Input: part model. Units: mm. Frame: model coordinates. Face numbers are marked on the shaded views. A direction names the side the tool comes from. Give positions to 0.01 mm unless a question says otherwise; leave off trailing zeros. Loops run counter-clockwise (first coordinate to the right, second up) from the corner with the lowest first, then second, coordinate; pieces in that order, holes last. Notation, with made-up numbers: (68.5, 24.25) - (73.5, 24.25) arc R28 ccw to (73.5, 56.25) - close; hole circle Ø1 at (44, 19). An arc over 180 degrees is marked (long way). One line per item, written item: value.
from build123d import *
from build123d.topology import SkipClean

# Parameters (mm, degrees)
SKETCH1_R                                           = 12
SKETCH1_R_2                                         = 2
SQUARE_BODY_DEPTH                                   = 11
CBORE_FOR_0_BINDING_HEAD_MACHINE_SCREW1_D           = 1.778
CBORE_FOR_0_BINDING_HEAD_MACHINE_SCREW1_CBORE_D     = 3.97002
CBORE_FOR_0_BINDING_HEAD_MACHINE_SCREW1_CBORE_DEPTH = 4.812792
CBORE_FOR_0_BINDING_HEAD_MACHINE_SC_2_D             = 1.778
CBORE_FOR_0_BINDING_HEAD_MACHINE_SC_2_CBORE_D       = 3.97002
CBORE_FOR_0_BINDING_HEAD_MACHINE_SC_2_CBORE_DEPTH   = 4.812792
F_6_32_TAPPED_HOLE2_D                               = 2.7051
F_6_32_TAPPED_HOLE2_DEPTH                           = 10.5
CENTER_SPINDLE_DEPTH                                = 21.223748416
SKETCH1_3_R                                         = 14
SKETCH1_3_R_2                                       = 12
TOP_FLANGE_DEPTH                                    = 2
BOTTOM_START                                        = 9
SKETCH1_4_R                                         = 14
SKETCH1_4_R_2                                       = 12
BOTTOM_FLANGE_DEPTH                                 = 2


with BuildPart() as part:
    # Sketch1 → Square Body (new body)
    # profile 1 of 10: a face of its own
    with BuildSketch(Plane.XY):
        Circle(SKETCH1_R)
        Circle(SKETCH1_R_2, mode=Mode.SUBTRACT)
    # profile 2 of 10: a face of its own
    with BuildSketch(Plane.XY):
        with BuildLine():
            Line((-12, 7.211102551), (-12, 0))
            ThreePointArc((-12, 0), (-8.485281374, 8.485281374), (0, 12))
            Line((0, 12), (-7.211102551, 12))
            ThreePointArc((-7.211102551, 12), (-9.899494937, 9.899494937), (-12, 7.211102551))
        make_face()
    # profile 3 of 10: a face of its own
    with BuildSketch(Plane.XY):
        with BuildLine():
            Line((-12, 12), (-12, 7.211102551))
            ThreePointArc((-12, 7.211102551), (-9.899494937, 9.899494937), (-7.211102551, 12))
            Line((-7.211102551, 12), (-12, 12))
        make_face()
    # profile 4 of 10: a face of its own
    with BuildSketch(Plane.XY):
        with BuildLine():
            ThreePointArc((0, -12), (-8.485281374, -8.485281374), (-12, 0))
            Line((-12, 0), (-12, -7.211102551))
            ThreePointArc((-12, -7.211102551), (-9.899494937, -9.899494937), (-7.211102551, -12))
            Line((-7.211102551, -12), (0, -12))
        make_face()
    # profile 5 of 10: a face of its own
    with BuildSketch(Plane.XY):
        with BuildLine():
            ThreePointArc((-7.211102551, -12), (-9.899494937, -9.899494937), (-12, -7.211102551))
            Line((-12, -7.211102551), (-12, -12))
            Line((-12, -12), (-7.211102551, -12))
        make_face()
    # profile 6 of 10: a face of its own
    with BuildSketch(Plane.XY):
        with BuildLine():
            ThreePointArc((12, 0), (8.485281374, -8.485281374), (0, -12))
            Line((0, -12), (7.211102551, -12))
            ThreePointArc((7.211102551, -12), (9.899494937, -9.899494937), (12, -7.211102551))
            Line((12, -7.211102551), (12, 0))
        make_face()
    # profile 7 of 10: a face of its own
    with BuildSketch(Plane.XY):
        with BuildLine():
            ThreePointArc((12, -7.211102551), (9.899494937, -9.899494937), (7.211102551, -12))
            Line((7.211102551, -12), (12, -12))
            Line((12, -12), (12, -7.211102551))
        make_face()
    # profile 8 of 10: a face of its own
    with BuildSketch(Plane.XY):
        with BuildLine():
            Line((7.211102551, 12), (0, 12))
            ThreePointArc((0, 12), (8.485281374, 8.485281374), (12, 0))
            Line((12, 0), (12, 7.211102551))
            ThreePointArc((12, 7.211102551), (9.899494937, 9.899494937), (7.211102551, 12))
        make_face()
    # profile 9 of 10: a face of its own
    with BuildSketch(Plane.XY):
        with BuildLine():
            Line((12, 12), (7.211102551, 12))
            ThreePointArc((7.211102551, 12), (9.899494937, 9.899494937), (12, 7.211102551))
            Line((12, 7.211102551), (12, 12))
        make_face()
    # profile 10 of 10: a face of its own
    with BuildSketch(Plane.XY):
        with BuildLine():
            ThreePointArc((2, 0), (1.870828693, 0.707106781), (1.5, 1.322875656))
            Line((1.5, 1.322875656), (1.5, -1.322875656))
            ThreePointArc((1.5, -1.322875656), (1.870828693, -0.707106781), (2, 0))
        make_face()
    extrude(amount=SQUARE_BODY_DEPTH)

    # CBORE for #0 Binding Head Machine Screw1 (through all)
    with Locations(Plane(origin=(-12, 7.5, 5.85), x_dir=(0, -1, 0), z_dir=(-1, 0, 0))):
        with Locations((0, 0)):
            CounterBoreHole(CBORE_FOR_0_BINDING_HEAD_MACHINE_SCREW1_D / 2, CBORE_FOR_0_BINDING_HEAD_MACHINE_SCREW1_CBORE_D / 2, CBORE_FOR_0_BINDING_HEAD_MACHINE_SCREW1_CBORE_DEPTH)

    # CBORE for _0 Binding Head Machine Sc 2 (through all)
    with Locations(Plane(origin=(12, -7.5, 5.85), x_dir=(0, 0, 1), z_dir=(1, 0, 0))):
        with Locations((0, 0)):
            CounterBoreHole(CBORE_FOR_0_BINDING_HEAD_MACHINE_SC_2_D / 2, CBORE_FOR_0_BINDING_HEAD_MACHINE_SC_2_CBORE_D / 2, CBORE_FOR_0_BINDING_HEAD_MACHINE_SC_2_CBORE_DEPTH)

    # #6-32 Tapped Hole2
    with Locations(Plane(origin=(12, 0, 5.85), x_dir=(0, 1, 0), z_dir=(1, 0, 0))):
        with Locations((0, 0)):
            Hole(F_6_32_TAPPED_HOLE2_D / 2, depth=F_6_32_TAPPED_HOLE2_DEPTH)

    # Sketch1<5> → Center Spindle (cut, through all)
    with SkipClean():  # the faces are left unmerged after this step: merging them gives an invalid solid
        with BuildSketch(Plane.XY):
            with BuildLine():
                ThreePointArc((0, -12), (-8.485281374, -8.485281374), (-12, 0))
                Line((-12, 0), (-12, -7.211102551))
                ThreePointArc((-12, -7.211102551), (-9.899494937, -9.899494937), (-7.211102551, -12))
                Line((-7.211102551, -12), (0, -12))
            make_face()
            with BuildLine():
                ThreePointArc((-7.211102551, -12), (-9.899494937, -9.899494937), (-12, -7.211102551))
                Line((-12, -7.211102551), (-12, -12))
                Line((-12, -12), (-7.211102551, -12))
            make_face()
            with BuildLine():
                Line((-12, 7.211102551), (-12, 0))
                ThreePointArc((-12, 0), (-8.485281374, 8.485281374), (0, 12))
                Line((0, 12), (-7.211102551, 12))
                ThreePointArc((-7.211102551, 12), (-9.899494937, 9.899494937), (-12, 7.211102551))
            make_face()
            with BuildLine():
                Line((-12, 12), (-12, 7.211102551))
                ThreePointArc((-12, 7.211102551), (-9.899494937, 9.899494937), (-7.211102551, 12))
                Line((-7.211102551, 12), (-12, 12))
            make_face()
            with BuildLine():
                Line((7.211102551, 12), (0, 12))
                ThreePointArc((0, 12), (8.485281374, 8.485281374), (12, 0))
                Line((12, 0), (12, 7.211102551))
                ThreePointArc((12, 7.211102551), (9.899494937, 9.899494937), (7.211102551, 12))
            make_face()
            with BuildLine():
                Line((12, 12), (7.211102551, 12))
                ThreePointArc((7.211102551, 12), (9.899494937, 9.899494937), (12, 7.211102551))
                Line((12, 7.211102551), (12, 12))
            make_face()
            with BuildLine():
                ThreePointArc((12, 0), (8.485281374, -8.485281374), (0, -12))
                Line((0, -12), (7.211102551, -12))
                ThreePointArc((7.211102551, -12), (9.899494937, -9.899494937), (12, -7.211102551))
                Line((12, -7.211102551), (12, 0))
            make_face()
            with BuildLine():
                ThreePointArc((12, -7.211102551), (9.899494937, -9.899494937), (7.211102551, -12))
                Line((7.211102551, -12), (12, -12))
                Line((12, -12), (12, -7.211102551))
            make_face()
        extrude(amount=CENTER_SPINDLE_DEPTH, mode=Mode.SUBTRACT)

    # Sketch1<3> → Top Flange (add)
    with SkipClean():  # the faces are left unmerged after this step: merging them gives an invalid solid
        with BuildSketch(Plane.XY):
            Circle(SKETCH1_3_R)
            Circle(SKETCH1_3_R_2, mode=Mode.SUBTRACT)
        extrude(amount=TOP_FLANGE_DEPTH)

    # Sketch1<4> → Bottom Flange (add)
    with SkipClean():  # the faces are left unmerged after this step: merging them gives an invalid solid
        with BuildSketch(Plane.XY.offset(BOTTOM_START)):
            Circle(SKETCH1_4_R)
            Circle(SKETCH1_4_R_2, mode=Mode.SUBTRACT)
        extrude(amount=BOTTOM_FLANGE_DEPTH)


solid = part.part
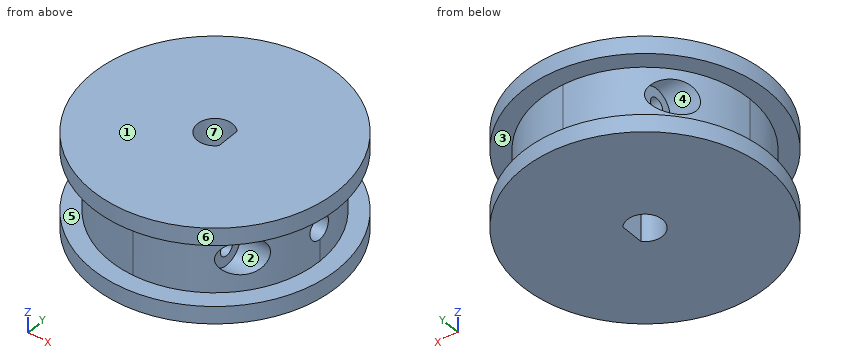
Item 1: Draft query along X for the marked faces 5, 6 and 7. Return one class per face: pulls with the +X half, pulls with the -X half, needs draft (parallel to the pull), parting line crosses it, or undercut.
Verdict:
face 5: needs draft
face 6: parting line crosses it
face 7: undercut
Item 2: Access query for the marked faces 1, 2, 3 and 4. Directions: +Z, -Z, +X, -X, +Y, -Y. A direction counts if a zero-diameter tool reaches every point of the face in a straight line with its end or side. Return the directions, or none.
Verdict:
face 1: +Z, +X, -X, +Y, -Y
face 2: +X
face 3: none
face 4: -X
Item 3: Section D-D, the plane z = 3. Output: boundary loops of the cut face in (x, y).
Verdict:
outline: circle Ø24 at (0, 0); hole (1.5, -1.32) - (1.5, 1.32) arc R2 ccw (long way) to start
Item 4: Pin query (flat end, axial travel): P1, Ø6, axis at y = -5.5, z = 4.5, coming from the -X side; P2, Ø5, axis at y = 7.5, z = 5.85, coming from the -X side; P3, Ø2.5, axis at y = -7.5, z = 5.85, coming from the +X side; P4, Ø1.6, axis at y = 7.5, z = 5.85, coming from the -X side. Return the tip coordinate at first contact, or that it passes through.
Verdict:
P1: stops at x = -13.46
P2: stops at x = -10.91
P3: stops at x = 7.19
P4: passes through
Item 5: Section C-C, the plane x = 5.5. Output: boundary loops of the cut face in (y, z), and give its area (3 significant figures).
Verdict:
outline: (-12.87, 0) - (12.87, 0) - (12.87, 2) - (10.67, 2) - (10.67, 9) - (12.87, 9) - (12.87, 11) - (-12.87, 11) - (-12.87, 9) - (-10.67, 9) - (-10.67, 2) - (-12.87, 2) - close; hole circle Ø1.78 at (-7.5, 5.85); hole circle Ø2.71 at (0, 5.85); hole circle Ø1.78 at (7.5, 5.85)
area: 242 mm^2
Item 6: Section B-B, the plane x = -5. Output: boundary loops of the cut face in (y, z), and give its area (3 significant figures).
Verdict:
outline: (-13.08, 0) - (13.08, 0) - (13.08, 2) - (10.91, 2) - (10.91, 9) - (13.08, 9) - (13.08, 11) - (-13.08, 11) - (-13.08, 9) - (-10.91, 9) - (-10.91, 2) - (-13.08, 2) - close; hole circle Ø1.78 at (-7.5, 5.85); hole circle Ø1.78 at (7.5, 5.85)
area: 252 mm^2
Item 7: Material intervals for L1, parallel to Z at x = -12, y = 2.25; L2, parallel to Z at x = -2, y = 7.5; L3, parallel to Y at x = 6.25, z = 5.85, sorted ascending.
Verdict:
L1: z = 0 to 2, 9 to 11
L2: z = 0 to 4.96, 6.74 to 11
L3: y = -10.24 to -8.39, -6.61 to -1.35, 1.35 to 6.61, 8.39 to 10.24
Item 8: Section A-A, the plane y = 7.5. Output: boundary loops of the cut face in (x, z) (1 decimal).
Verdict:
outline: (-11.8, 0) - (11.8, 0) - (11.8, 2) - (9.4, 2) - (9.4, 5) - (-7.2, 5) - (-7.2, 3.9) - (-9.4, 3.9) - (-9.4, 2) - (-11.8, 2) - close; (-11.8, 9) - (-9.4, 9) - (-9.4, 7.8) - (-7.2, 7.8) - (-7.2, 6.7) - (9.4, 6.7) - (9.4, 9) - (11.8, 9) - (11.8, 11) - (-11.8, 11) - close
